Verification items for this drawing (mm, ordinates from the low corner). Round coordinates to 2 decimals unless told otherwise and drop trailing zeros. Order: outer loops, then holes, each group sorted by start corner. A loop starts at its lowest first (then second) coordinate and runs counter-clockwise, first axis right, second up. Notation, with made-up numbers: (83.5, 18.25) -> (121.5, 18.25) arc R24 ccw to (121.5, 28.25) -> close; hole circle Ø3 at (2, 50.5). An arc over 180 degrees is marked (long way). Return JSON: item names as keys, results as strings. Group by question number.
Item 1: Scan lines: probe 1 along X at (y, z) = (1.9, 57.15) (1 decimal); probe 2 along X at (y, z) = (0.9, 37); probe 3 along Z at (x, y) = (14, 3.2) (1 decimal). Record each from-to range of solid material in increasing order. Write a range as from..to.
Item 2: Sectioned sample at A-A on x = 57.15. Give the number of separate pieces and of enclosed holes in the cut face.
Item 3: Sectioned sample at C-C on x = 72.5. Record the cut outline in (y, z) (1 decimal).
Item 4: Depth check by flat-ended pin: pin 1 Ø5 at (x, z) = (98.39, 33.34) entering from -Y. Enter the tip coordinate at first touch or a pass-through.
Item 5: Sectioned sample at B-B on z = 57.15. Record the cut outline in (x, y) (1 decimal), plus the area to 3 significant figures.
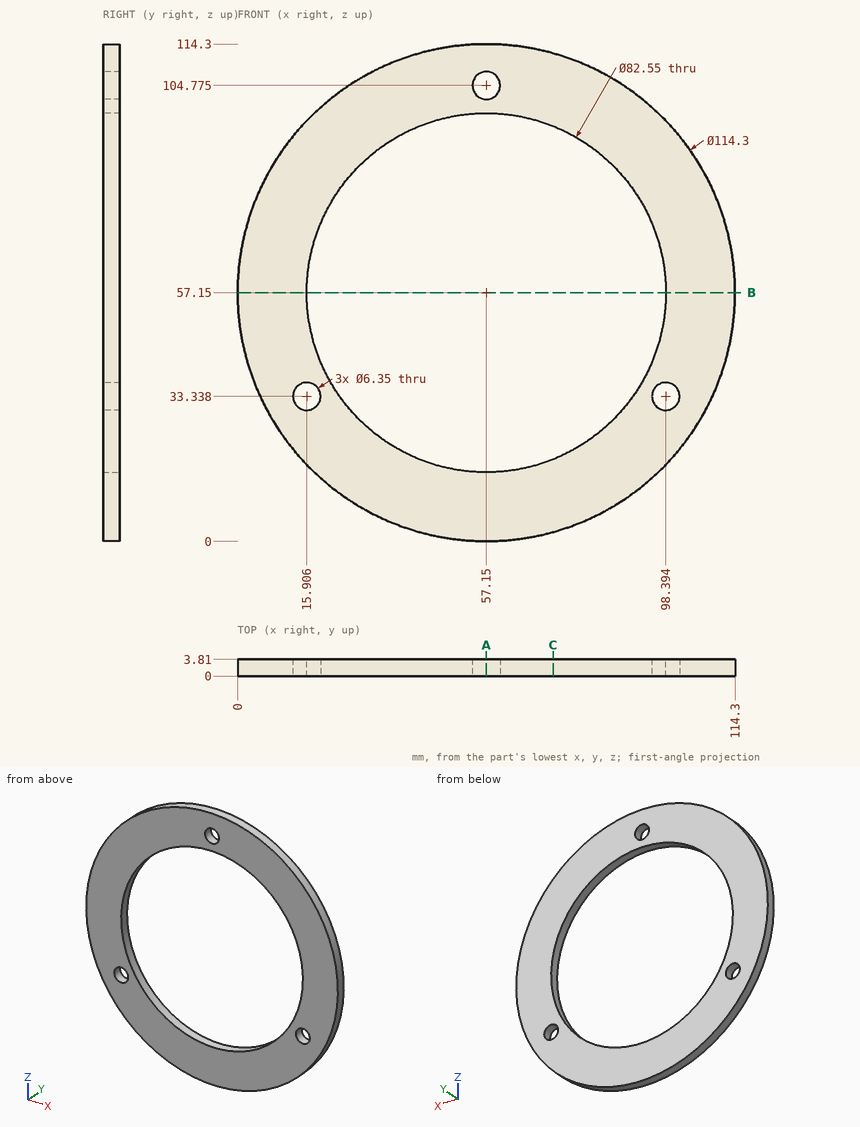
Recorded:
{
 "1": {"probe 1": "0..15.9, 98.4..114.3", "probe 2": "3.67..21.13, 93.17..110.63", "probe 3": "19.7..30.8, 35.9..94.6"},
 "2": {"separate pieces": "3", "enclosed holes": "0"},
 "3": {"outline": "(0, 2.1) -> (3.8, 2.1) -> (3.8, 18.8) -> (0, 18.8) -> close; (0, 95.5) -> (3.8, 95.5) -> (3.8, 112.2) -> (0, 112.2) -> close"},
 "4": {"pin 1": "through"},
 "5": {"outline": "(0, 0) -> (15.9, 0) -> (15.9, 3.8) -> (0, 3.8) -> close; (98.4, 0) -> (114.3, 0) -> (114.3, 3.8) -> (98.4, 3.8) -> close", "area": "121 mm²"}
}
